Verification items for the finished model (mm, model axes). Face numbers are marked on the shaded views. A direction names the side the tool comes from. Give positions to 0.01 mm unless a question says otherwise; leave off trailing zeros. Loops run counter-clockwise (first coordinate to the right, second up) from the corner with the lowest first, then second, coordinate; pieces in that order, holes last. Notation, with made-up numbers: M -36.5,25.25 L -15.5,25.25 A24 ccw -15.5,38.25 Z; hole C 19.5,33.25 d6. An arc over 180 degrees is marked long. Use CSV: the item, a comma, the result in double quotes.
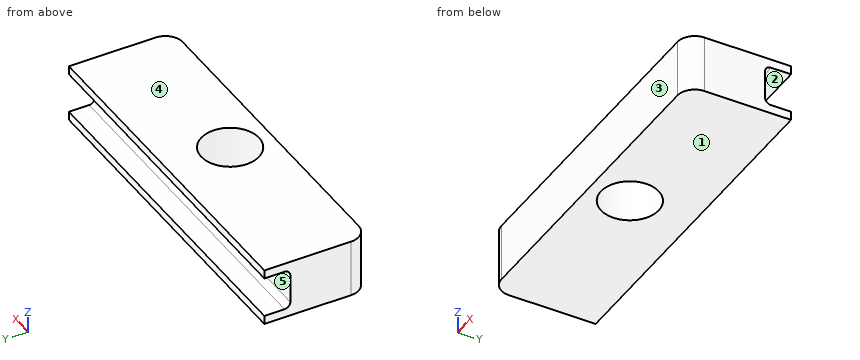
from build123d import *

# Parameters (mm, degrees)
F0_W     = 60
F0_H     = 18
F0_R     = 5
F1_DEPTH = 10
F2_R     = 3
F3_W     = 60
F3_H     = 7
F4_DEPTH = 4.5
F5_R     = 1


with BuildPart() as f1:
    # F0 (on Top) → F1 (new body)
    with BuildSketch(Plane.XY):
        with Locations((0, -9)):
            Rectangle(F0_W, F0_H)
        with Locations((0, -11)):
            Circle(F0_R, mode=Mode.SUBTRACT)
    extrude(amount=F1_DEPTH)

    # F2
    f2_edges = [f1.edges().sort_by_distance(p)[0] for p in [
        (-30, -18, 5),
        (30, -18, 5),
    ]]
    fillet(f2_edges, radius=F2_R)

    # F3 (on face) → F4 (cut)
    with BuildSketch(Plane(origin=(0, 0, 0), x_dir=(-1, 0, 0), z_dir=(0, 1, 0))):
        with Locations((0, 5)):
            Rectangle(F3_W, F3_H)
    extrude(amount=-F4_DEPTH, mode=Mode.SUBTRACT)

    # F5
    f5_edges = [f1.edges().sort_by_distance(p)[0] for p in [
        (0, -4.5, 8.5),
        (0, -4.5, 1.5),
    ]]
    fillet(f5_edges, radius=F5_R)


solid = f1.part
(1) Section check D-D on x = 12. Record the cut outline in (y, z).
Calculated:
outline,"M -18,0 L 0,0 L 0,1.5 L -3.5,1.5 A1 cw -4.5,2.5 L -4.5,7.5 A1 cw -3.5,8.5 L 0,8.5 L 0,10 L -18,10 Z"
(2) Mould release check, pull along Z, two halves, no side actions. Record for the marked faces 1, 2 and 3: released by +Z, released by -Z, zero draft, split by the parting line, or undercut.
Calculated:
face 1,"released by -Z"
face 2,"undercut"
face 3,"zero draft"
(3) Section check B-B on y = -11. Record the cut outline in (x, z), plus the area to 3 significant figures.
Calculated:
outline,"M -30,0 L -5,0 L -5,10 L -30,10 Z; M 5,0 L 30,0 L 30,10 L 5,10 Z"
area,"500 mm²"
(4) Tool access check on the marked faces 4 and 5. Record the directions out of +Z, -Z, +X, -X, +Y, -Y that give a thin tool (end or side, any length) a straight path to the whole face; none if there is none.
Calculated:
face 4,"+Z, +X, -X, +Y, -Y"
face 5,"+X, -X, +Y"
(5) Section check C-C on z = 5.5. Record the cut outline in (x, y), plus the area to 3 significant figures.
Calculated:
outline,"M -30,-15 A3 ccw -27,-18 L 27,-18 A3 ccw 30,-15 L 30,-4.5 L -30,-4.5 Z; hole C 0,-11 d10"
area,"728 mm²"
(6) Depth check by flat-ended pin: pin 1 Ø10 at (x, y) = (16.5, -4) entering from -Z; pin 2 Ø2.5 at (x, z) = (1, 5.5) entering from +Y. Enter the tip coordinate at first touch or a pass-through.
Calculated:
pin 1,"stops at z = 0"
pin 2,"stops at y = -4.5"
(7) Section check A-A on x = 3. Record the cut outline in (y, z).
Calculated:
outline,"M -18,0 L -15,0 L -15,10 L -18,10 Z; M -7,0 L 0,0 L 0,1.5 L -3.5,1.5 A1 cw -4.5,2.5 L -4.5,7.5 A1 cw -3.5,8.5 L 0,8.5 L 0,10 L -7,10 Z"
(8) Scan lines: L1, parallel to Y at x = 0, z = 6; L2, parallel to Z at x = 27.5, y = -3.25; L3, parallel to Y at x = -24, z = 6. Record each from-to range of solid material in increasing order. Write a range as from..to.
Calculated:
L1,"y = -18..-16, -6..-4.5"
L2,"z = 0..1.5, 8.5..10"
L3,"y = -18..-4.5"
